Input: part model. Units: mm. Frame: model coordinates. A direction names the side the tool comes from. Round coordinates to 2 decimals unless told otherwise and drop trailing zeros. Loops run counter-clockwise (first coordinate to the right, second up) from the corner with the lowest first, then second, coordinate; pieces in that order, holes last. Notation, with made-up numbers: (9.5, -25.75) - (52.5, -25.75) arc R17 cw to (52.5, -20.75) - close; hole circle Ø6 at (-27, 74). An arc over 180 degrees is marked (long way). Write each question's results on one line, items separated by ' | '.
from build123d import *

# Parameters (mm, degrees)
EXTRUDE_THIN1_DEPTH = 317.5
FILLET1_R           = 1.27


with BuildPart() as part:
    # Sketch1 → Extrude-Thin1 (new body)
    with BuildSketch(Plane.XY):
        Polygon((0, 4.7625), (0, 1.5875), (-17.4625, 0), (-7.9375, 31.75), (-7.9375, 38.1), (-3.175, 38.1), (-3.175, 30.1625), (-4.445, 30.1625), (-4.445, 36.83), (-6.6675, 36.83), (-6.6675, 31.563603578), (-15.706108342, 1.434909105), (-1.27, 2.74728259), (-1.27, 4.7625), align=None)
    extrude(amount=-EXTRUDE_THIN1_DEPTH)

    # Fillet1
    fillet1_edges = [part.edges().sort_by_distance(p)[0] for p in [
        (-6.6675, 31.563603578, -158.75),
        (0, 1.5875, -158.75),
        (-17.4625, 0, -158.75),
        (-7.9375, 38.1, -158.75),
        (-3.175, 38.1, -158.75),
    ]]
    fillet(fillet1_edges, radius=FILLET1_R)


solid = part.part
1. Line query: line 1 (X direction, y = 36, z = -176) (1 decimal); line 2 (X direction, y = 3, z = -219.5); line 3 (Y direction, x = -1.75, z = -77). Output: solid intervals per line, ascending. Write a range as [from, to].
Answer:
line 1: [-7.9, -6.7], [-4.4, -3.2] | line 2: [-16.56, -15.24], [-1.27, 0] | line 3: [1.43, 2.7]
2. Set-up query: faces 1 (the flat face through (-4.445, 33, -157)), 2 (the flat face through (-7.938, 34, -157)), 3 (the flat face through (-11, 18, -317.5)). Return all of +Z, -Z, +X, -X, +Y, -Y with unobstructed straight access to the full face (end or side cutting, diameter ignored); none if empty.
Answer:
face 1: +Z, -Z | face 2: +Z, -Z, -X, +Y | face 3: -Z, +X, -X, +Y, -Y
3. Mould query, pull axis Y, two halves, no side actions, for faces 4 (the flat face through (-11.15, 16.62, -156.53)), 5 (the flat face through (-3.175, 34, -157)), 6 (the flat face through (-12.49, 16.57, -156.53)). Classes: pulls with the +Y half, pulls with the -Y half, needs draft (parallel to the pull), parting line crosses it, or undercut.
Answer:
face 4: undercut | face 5: needs draft | face 6: pulls with the +Y half
4. Section query C-C, the plane y = 22.5. Output: boundary loops of the cut face in (x, z), plus the area to 3 significant figures.
Answer:
outline: (-10.71, -317.5) - (-9.39, -317.5) - (-9.39, 0) - (-10.71, 0) - close | area: 421 mm^2
5. Section query A-A, the plane x = -12. Output: boundary loops of the cut face in (y, z), plus the area to 3 significant figures.
Answer:
outline: (0.5, -317.5) - (1.77, -317.5) - (1.77, 0) - (0.5, 0) - close; (13.79, -317.5) - (18.21, -317.5) - (18.21, 0) - (13.79, 0) - close | area: 1,810 mm^2
6. Contact query for flat-ended pins moving along their axis: pin 1 (5.5 mm diameter, centred on y = 35, z = -209.5, fed in from +X) (3 decimals); pin 2 (3 mm diameter, centred on x = -2.5, z = -268, fed in from -Y); pin 3 (1.8 mm diameter, centred on x = -6, z = -217.5, fed in from -Y). Output: stop coordinate, or through.
Answer:
pin 1: x = -3.175 | pin 2: y = 1.22 | pin 3: y = 0.96
